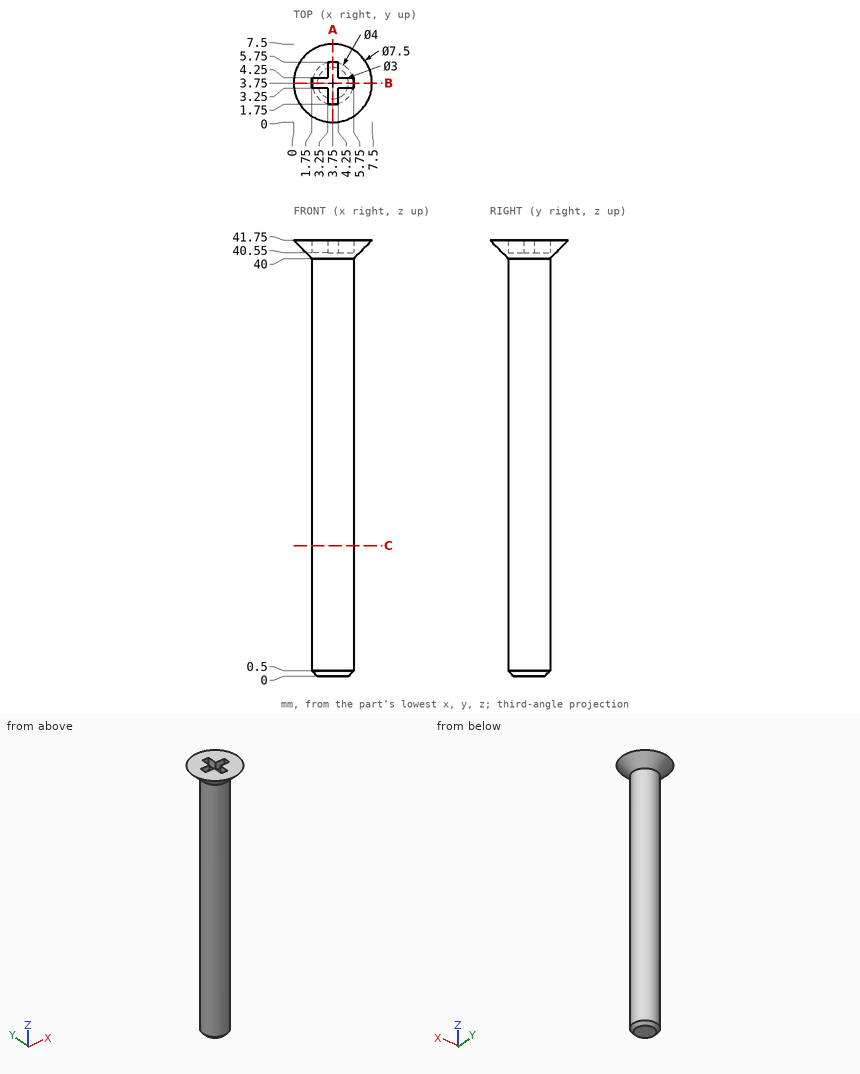
Part print with two shaded views. Sizes in mm from the minimum x, y, z corner. Give positions to 0.01 mm unless a question says otherwise; leave off trailing zeros. Order: outer loops, then holes, each group sorted by start corner. A loop starts at its lowest first (then second) coordinate and runs counter-clockwise, first axis right, second up. Notation, with made-up numbers: (-23, -26) - (-14, -26) arc R15 ccw to (-14, -15) - close; hole circle Ø2 at (36.5, 67.5). An arc over 180 degrees is marked (long way). Write each question's results on one line, items separated by ' | '.
1. Pin check, flat tips, straight feed: pin 1 (1.5 mm diameter, centred on y = 3, z = 7.5, fed in from +X); pin 2 (0.6 mm diameter, centred on y = 2.5, z = 41, fed in from -X); pin 3 (1 mm diameter, centred on x = 5, z = 41.5, fed in from -Y). Stop position of each tip, or through.
Calculated:
pin 1: stops at x = 5.75 | pin 2: stops at x = 0.68 | pin 3: stops at y = 0.09
2. Saw through at A-A on x = 3.75. List the corners of the cut face in (y, z), and give its area (3 significant figures).
Calculated:
outline: (0, 41.75) - (1.75, 40) - (1.75, 0.5) - (2.25, 0) - (5.25, 0) - (5.75, 0.5) - (5.75, 40) - (7.5, 41.75) - (5.75, 41.75) - (5.75, 40.55) - (1.75, 40.55) - (1.75, 41.75) - close | area: 165 mm2
3. Saw through at C-C on z = 12.5. List the corners of the cut face in (x, y).
Calculated:
outline: circle Ø4 at (3.75, 3.75)
4. Probe L1, parallel to Z at x = 6.5, y = 2.25; L2, parallel to Y at x = 3.25, z = 35; L3, parallel to Z at x = 2.5, y = 5.75. List the from-to ranges inside material, lowest first. Write a range as from..to.
Calculated:
L1: z = 41.13..41.75 | L2: y = 1.81..5.69 | L3: z = 40.36..41.75
